```python
from build123d import *

# Parameters (mm, degrees)
SKETCH1_R           = 9
BOSS_EXTRUDE1_DEPTH = 30
SKETCH3_R           = 2.5
CUT_EXTRUDE1_DEPTH  = 17.65


with BuildPart() as part:
    # Sketch1 → Boss-Extrude1 (new body)
    with BuildSketch(Plane.XY):
        with BuildLine():
            Line((0, 0), (-25, 0))
            Line((-25, 0), (-25, 10))
            Line((-25, 10), (-15, 10))
            ThreePointArc((-15, 10), (-13.232233047, 10.732233047), (-12.5, 12.5))
            Line((-12.5, 12.5), (-12.5, 14.5))
            ThreePointArc((-12.5, 14.5), (0, 27), (12.5, 14.5))
            Line((12.5, 14.5), (12.5, 12.5))
            ThreePointArc((12.5, 12.5), (13.232233047, 10.732233047), (15, 10))
            Line((15, 10), (25, 10))
            Line((25, 10), (25, 0))
            Line((25, 0), (0, 0))
        make_face()
        with Locations((0, 14.5)):
            Circle(SKETCH1_R, mode=Mode.SUBTRACT)
    extrude(amount=BOSS_EXTRUDE1_DEPTH)

    # Sketch3 → Cut-Extrude1 (cut)
    with BuildSketch(Plane(origin=(0, 10, 0), x_dir=(1, 0, 0), z_dir=(0, 1, 0))):
        with Locations(Location((-20, -7.5, 0), (0, 0, 270))):
            Circle(SKETCH3_R)
        with Locations(Location((-20, -22.5, 0), (0, 0, 180))):
            Circle(SKETCH3_R)
        with Locations(Location((20, -22.5, 0), (0, 0, 270))):
            Circle(SKETCH3_R)
        with Locations(Location((20, -7.5, 0), (0, 0, 180))):
            Circle(SKETCH3_R)
    extrude(amount=-CUT_EXTRUDE1_DEPTH, mode=Mode.SUBTRACT)


solid = part.part
```
Here's how the part is built. I have some questions about the finished solid (model axes, mm). A direction names the side the tool comes from. Coordinates: 2 decimals unless noted, no trailing zeros. Write each loop counter-clockwise with the first axis right and the second up, starting at its lowest first coordinate (ties: lowest second). Pieces come first, ordered by that corner, then holes. Notation, with made-up numbers: M 11,43.25 L 43,43.25 A30 ccw 43,76.25 Z; hole C 84,77.25 d10. An arc over 180 degrees is marked long. Answer as CSV lines item,"result". Start each with the question number.
Q1. If we mould it in two halves opening along Z, with no side actions, what happens to faces 1 (the flat face through (0, 5, 30)), 2 (the cylindrical face through (22, 5, 21)), 3 (the flat face through (20, 10, 15))? For each: pulls with the +Z half, pulls with the -Z half, needs draft (parallel to the pull), parting line crosses it, or undercut.
Q2. Suppose I cut it at D-D, the plane y = 6.5. List the corners of the cut face in (x, z) for me.
Q3. Suppose I cut it at C-C, the plane x = -20. List the corners of the cut face in (y, z) for me.
Q4. For faces 4 (the flat face through (12.5, 14, 15)), 5 (the flat face through (-20, 10, 15)), 6 (the flat face through (-25, 5, 15)), which set-ups out of +Z, -Z, +X, -X, +Y, -Y let a thin tool reach every point of the face, with its end or its side?
Q5. Suppose I cut it at A-A, the plane z = 7.5. List the corners of the cut face in (x, y) for me.
Q6. Suppose I cut it at B-B, the plane x = 0. List the corners of the cut face in (y, z) for me, then the cut area to 3 significant figures.
Q7. Will these pins go through, and if not, where does the flat tip stop? pin 1 Ø1.6 at (y, z) = (13.5, 21.5) entering from -X; pin 2 Ø2 at (y, z) = (14, 20.5) entering from +X; pin 3 Ø6 at (x, z) = (-20, 22.5) entering from +Y; pin 4 Ø4.5 at (x, z) = (-20, 7.5) entering from -Y.
Q8. I need wall thicknesses on probe 1 along Y at (x, z) = (0, 20); probe 2 along Y at (x, z) = (-17.5, 5.5); probe 3 along X at (y, z) = (17.75, 6.75). Which ranges of each line are inside material? Lowest first, please. Write a range as [from, to].
Entries:
1,face 1,"pulls with the +Z half"
1,face 2,"undercut"
1,face 3,"needs draft"
2,outline,"M -25,0 L -4.12,0 L -4.12,30 L -25,30 Z; M 4.12,0 L 25,0 L 25,30 L 4.12,30 Z; hole C -20,7.5 d5; hole C -20,22.5 d5; hole C 20,7.5 d5; hole C 20,22.5 d5"
3,outline,"M 0,0 L 10,0 L 10,5 L 0,5 Z; M 0,10 L 10,10 L 10,20 L 0,20 Z; M 0,25 L 10,25 L 10,30 L 0,30 Z"
4,face 4,"+Z, -Z, +X, +Y"
4,face 5,"+Z, -Z, -X, +Y"
4,face 6,"+Z, -Z, -X, +Y, -Y"
5,outline,"M -25,0 L -22.5,0 L -22.5,10 L -25,10 Z; M -17.5,0 L 17.5,0 L 17.5,10 L 15,10 A2.5 cw 12.5,12.5 L 12.5,14.5 A12.5 ccw -12.5,14.5 L -12.5,12.5 A2.5 cw -15,10 L -17.5,10 Z; M 22.5,0 L 25,0 L 25,10 L 22.5,10 Z; hole C 0,14.5 d18"
6,outline,"M 0,0 L 5.5,0 L 5.5,30 L 0,30 Z; M 23.5,0 L 27,0 L 27,30 L 23.5,30 Z"
6,area,"270 mm²"
7,pin 1,"stops at x = -12.5"
7,pin 2,"stops at x = 12.5"
7,pin 3,"stops at y = 10"
7,pin 4,"passes through"
8,probe 1,"y = [0, 5.5], [23.5, 27]"
8,probe 2,"y = [0, 10]"
8,probe 3,"x = [-12.07, -8.39], [8.39, 12.07]"
